Verification items for the finished model (mm, model axes). Face numbers are marked on the shaded views. A direction names the side the tool comes from. Round coordinates to 2 decimals unless told otherwise and drop trailing zeros. Order: outer loops, then holes, each group sorted by start corner. A loop starts at its lowest first (then second) coordinate and runs counter-clockwise, first axis right, second up. Notation, with made-up numbers: M 25.5,11 L 33.5,11 A17 ccw 33.5,36 Z; hole C 46.5,74 d5. An arc over 180 degrees is marked long. Use one line per item in the form item = value. Start each with the question number.
Item 1: Tool access check on the marked faces 1 and 2. Record the directions out of +Z, -Z, +X, -X, +Y, -Y that give a thin tool (end or side, any length) a straight path to the whole face; none if there is none.
Item 2: Release check for a two-part mould opening along X. For the marked faces 3, 4 and 5 record: +X half, -X half, draft (parallel to the pull), parting line (faces both ways), or undercut.
Item 3: Cross-section at D-D on z = 115. Enter the section's corners in (x, y), then the cut area to 3 significant figures.
Item 4: Go/stop test with flat-tipped pins: pin 1 Ø12.5 at (y, z) = (23, 63) entering from +X; pin 2 Ø0.8 at (x, y) = (-3.5, 22.5) entering from +Z; pin 3 Ø6 at (x, z) = (2.5, 107.5) entering from +Y. Record where each tip stops, or that it passes through.
Item 5: Cross-section at C-C on y = 7.75. Enter the section's corners in (x, z), then the cut area to 3 significant figures.
Item 6: Cross-section at B-B on z = 2. Enter the section's corners in (x, y), then the cut area to 3 significant figures.
Item 7: Cross-section at A-A on x = -3.75. Enter the section's corners in (y, z), then the cut area to 3 significant figures.
Item 8: Thickness scan on probe 1 along Z at (x, y) = (-3.5, 14); probe 2 along X at (y, z) = (23.5, 2.5); probe 3 along Y at (x, z) = (4, 73). Record the ranges inside material, lowest first. Write a range as [from, to].
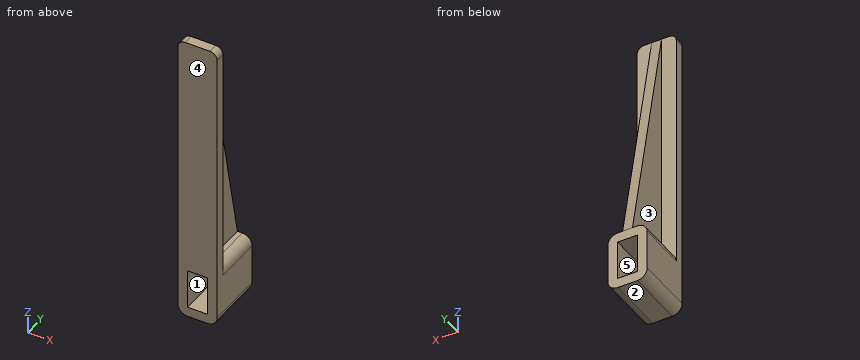
from build123d import *

# Parameters (mm, degrees)
SKETCH_1_W      = 20
SKETCH_1_H      = 30
SKETCH_1_W_2    = 10
SKETCH_1_H_2    = 20
EXTRUDE_1_DEPTH = 30
SKETCH_1_3_W    = 20
SKETCH_1_3_H    = 120
EXTRUDE_2_DEPTH = 5
RIB_1_REACH     = 140.654
SKETCH_2_WALL_W = 401.884999198
SKETCH_2_WALL_H = 5
FILLET_1_R      = 5
FILLET_3_R      = 3.75


with BuildPart() as part:
    # Эскиз1 → Бобышка-Вытянуть1 (new body)
    with BuildSketch(Plane(origin=(0, 0, 0), x_dir=(1, 0, 0), z_dir=(0, 1, 0))):
        Rectangle(SKETCH_1_W, SKETCH_1_H)
        Rectangle(SKETCH_1_W_2, SKETCH_1_H_2, mode=Mode.SUBTRACT)
    extrude(amount=EXTRUDE_1_DEPTH)

    # Эскиз1<3> → Бобышка-Вытянуть2 (add)
    with BuildSketch(Plane(origin=(0, 0, 0), x_dir=(1, 0, 0), z_dir=(0, 1, 0))):
        with Locations((0, -75)):
            Rectangle(SKETCH_1_3_W, SKETCH_1_3_H)
    extrude(amount=EXTRUDE_2_DEPTH)

    # Эскиз2 wall → Ребро1 (add, up to next)
    with BuildSketch(Plane(origin=(0, 17.5, 75), x_dir=(0, 0.203954254112, -0.978980419738), z_dir=(0, 0.978980419738, 0.203954254112)), mode=Mode.PRIVATE) as rib_1_sk1:
        Rectangle(SKETCH_2_WALL_W, SKETCH_2_WALL_H)
    rib_1_tool1 = extrude(rib_1_sk1.sketch, amount=-RIB_1_REACH, mode=Mode.PRIVATE) - part.part
    add(rib_1_tool1.solids().sort_by_distance((0, 17.5, 75))[0])

    # Скругление1
    fillet_1_edges = [part.edges().sort_by_distance(p)[0] for p in [
        (-10, 15, -15),
        (10, 15, -15),
        (10, 17.5, 15),
        (-10, 17.5, 15),
    ]]
    fillet(fillet_1_edges, radius=FILLET_1_R)

    # Скругление3
    fillet_3_edges = [part.edges().sort_by_distance(p)[0] for p in [
        (-10, 2.5, 135),
        (10, 2.5, 135),
    ]]
    fillet(fillet_3_edges, radius=FILLET_3_R)


solid = part.part
Output values:
q1.face_1 = +Y, -Y
q1.face_2 = -Z, +X, -X, +Y, -Y
q2.face_3 = -X half
q2.face_4 = draft
q2.face_5 = undercut
q3.outline = M -10,0 L 10,0 L 10,5 L 2.5,5 L 2.5,9.17 L -2.5,9.17 L -2.5,5 L -10,5 Z
q3.area = 121 mm2
q4.pin_1 = 2.5
q4.pin_2 = 15
q4.pin_3 = 11.35
q5.outline = M -10,-10 A5 ccw -5,-15 L 5,-15 A5 ccw 10,-10 L 10,10 A5 ccw 5,15 L 2.5,15 L 2.5,121.8 L -2.5,121.8 L -2.5,15 L -5,15 A5 ccw -10,10 Z; hole M -5,-10 L 5,-10 L 5,10 L -5,10 Z
q5.area = 913 mm2
q6.outline = M -10,0 L -5,0 L -5,30 L -10,30 Z; M 5,0 L 10,0 L 10,30 L 5,30 Z
q6.area = 300 mm2
q7.outline = M 0,-15 L 30,-15 L 30,-10 L 0,-10 Z; M 0,10 L 30,10 L 30,15 L 5,15 L 5,135 L 0,135 Z
q7.area = 900 mm2
q8.probe_1 = [-15, -10], [10, 15]
q8.probe_2 = [-10, -5], [5, 10]
q8.probe_3 = [0, 5]
